from build123d import *

# Parameters (mm, degrees)
SKETCH_1_W             = 50
SKETCH_1_H             = 136
EXTRUDE_1_DEPTH        = 2
SKETCH_3_R             = 1.525
CUT_EXTRUDE_1_DEPTH    = 10
CUT_EXTRUDE_2_DEPTH    = 22
PATTERN_LINEAR_1_COUNT = 5
PATTERN_LINEAR_1_PITCH = 14
MIRROR_2_COPY_1_DEPTH  = 22
MIRROR_2_COPY_2_DEPTH  = 22
MIRROR_2_COPY_3_DEPTH  = 22
MIRROR_2_COPY_4_DEPTH  = 22
MIRROR_2_COPY_5_DEPTH  = 22
FILLET_1_R             = 2


with BuildPart() as part:
    # 草图1 → 凸台-拉伸1 (new body)
    with BuildSketch(Plane.XY):
        Rectangle(SKETCH_1_W, SKETCH_1_H)
    extrude(amount=EXTRUDE_1_DEPTH)

    # 草图3 → 切除-拉伸1 (cut)
    with BuildSketch(Plane(origin=(0, 0, 0), x_dir=(-1, 0, 0), z_dir=(0, 0, -1))):
        with Locations((-13, 65)):
            Circle(SKETCH_3_R)
        with Locations((7, 65)):
            Circle(SKETCH_3_R)
    cut_extrude_1 = extrude(amount=-CUT_EXTRUDE_1_DEPTH, mode=Mode.SUBTRACT)

    # 镜向1: 切除-拉伸1 across plane
    add(cut_extrude_1.mirror(Plane.ZX), mode=Mode.SUBTRACT)

    # 草图4 → 切除-拉伸2 (cut)
    with BuildSketch(Plane(origin=(0, 0, 0), x_dir=(-1, 0, 0), z_dir=(0, 0, -1))):
        with BuildLine():
            Line((16, -5), (-16, -5))
            ThreePointArc((-16, -5), (-21, 0), (-16, 5))
            Line((-16, 5), (16, 5))
            ThreePointArc((16, 5), (21, 0), (16, -5))
        make_face()
    cut_extrude_2 = extrude(amount=-CUT_EXTRUDE_2_DEPTH, mode=Mode.SUBTRACT)

    # 阵列(线性)1: 切除-拉伸2 ×5
    with Locations(*[(0, -i * PATTERN_LINEAR_1_PITCH, 0) for i in range(1, PATTERN_LINEAR_1_COUNT)]):
        add(cut_extrude_2, mode=Mode.SUBTRACT)

    # 镜向2 copy 1 sketch → 镜向2 copy 1 (cut)
    with BuildSketch(Plane(origin=(0, 14, 0), x_dir=(-1, 0, 0), z_dir=(0, 0, -1))):
        with BuildLine():
            Line((16, 5), (-16, 5))
            ThreePointArc((-16, 5), (-21, 0), (-16, -5))
            Line((-16, -5), (16, -5))
            ThreePointArc((16, -5), (21, 0), (16, 5))
        make_face()
    extrude(amount=-MIRROR_2_COPY_1_DEPTH, mode=Mode.SUBTRACT)

    # 镜向2 copy 2 sketch → 镜向2 copy 2 (cut)
    with BuildSketch(Plane(origin=(0, 28, 0), x_dir=(-1, 0, 0), z_dir=(0, 0, -1))):
        with BuildLine():
            Line((16, 5), (-16, 5))
            ThreePointArc((-16, 5), (-21, 0), (-16, -5))
            Line((-16, -5), (16, -5))
            ThreePointArc((16, -5), (21, 0), (16, 5))
        make_face()
    extrude(amount=-MIRROR_2_COPY_2_DEPTH, mode=Mode.SUBTRACT)

    # 镜向2 copy 3 sketch → 镜向2 copy 3 (cut)
    with BuildSketch(Plane(origin=(0, 42, 0), x_dir=(-1, 0, 0), z_dir=(0, 0, -1))):
        with BuildLine():
            Line((16, 5), (-16, 5))
            ThreePointArc((-16, 5), (-21, 0), (-16, -5))
            Line((-16, -5), (16, -5))
            ThreePointArc((16, -5), (21, 0), (16, 5))
        make_face()
    extrude(amount=-MIRROR_2_COPY_3_DEPTH, mode=Mode.SUBTRACT)

    # 镜向2 copy 4 sketch → 镜向2 copy 4 (cut)
    with BuildSketch(Plane(origin=(0, 56, 0), x_dir=(-1, 0, 0), z_dir=(0, 0, -1))):
        with BuildLine():
            Line((16, 5), (-16, 5))
            ThreePointArc((-16, 5), (-21, 0), (-16, -5))
            Line((-16, -5), (16, -5))
            ThreePointArc((16, -5), (21, 0), (16, 5))
        make_face()
    extrude(amount=-MIRROR_2_COPY_4_DEPTH, mode=Mode.SUBTRACT)

    # 镜向2 copy 5 sketch → 镜向2 copy 5 (cut)
    with BuildSketch(Plane(origin=(0, 0, 0), x_dir=(-1, 0, 0), z_dir=(0, 0, -1))):
        with BuildLine():
            Line((16, 5), (-16, 5))
            ThreePointArc((-16, 5), (-21, 0), (-16, -5))
            Line((-16, -5), (16, -5))
            ThreePointArc((16, -5), (21, 0), (16, 5))
        make_face()
    extrude(amount=-MIRROR_2_COPY_5_DEPTH, mode=Mode.SUBTRACT)

    # 圆角1
    fillet_1_edges = [part.edges().sort_by_distance(p)[0] for p in [
        (25, -68, 1),
        (-25, -68, 1),
        (-25, 68, 1),
        (25, 68, 1),
    ]]
    fillet(fillet_1_edges, radius=FILLET_1_R)


solid = part.part
Geometry: final body of the model. Coordinates: model frame, mm. A direction names the side the tool comes from. Give positions to 0.01 mm unless a question says otherwise; leave off trailing zeros. Write each loop counter-clockwise with the first axis right and the second up, starting at its lowest first coordinate (ties: lowest second). Pieces come first, ordered by that corner, then holes.
(1) Ray query, line 1 (X direction, y = -65, z = 0.8) (3 decimals); line 2 (X direction, y = -14, z = 0.6); line 3 (X direction, y = -18, z = 0.5). Return the intervals inside material, ascending.
(2) Access query for faces 1 (the flat face through (-3.8, 5.4, 0)), 2 (the cylindrical face through (21, -28, 1)). Directions: +Z, -Z, +X, -X, +Y, -Y. A direction counts if a zero-diameter tool reaches every point of the face in a straight line with its end or side. Return the directions, or none.
(3) Cut plane B-B, the plane x = 13. Give the number of separate pieces and of enclosed holes in the cut face, then the cut area to 3 significant figures.
(4) Cut plane A-A, the plane y = -25. Return loops of the section in (x, z), then the cut area to 3 significant figures.
Values follow:
1. line 1: x = -25 to -8.525, -5.475 to 11.475, 14.525 to 25
1. line 2: x = -25 to -21, 21 to 25
1. line 3: x = -25 to -19, 19 to 25
2. face 1: -Z, +X, -X, +Y, -Y
2. face 2: +Z, -Z
3. separate pieces: 12
3. enclosed holes: 0
3. area: 79.8 mm2
4. outline: (-25, 0) - (-20, 0) - (-20, 2) - (-25, 2) - close; (20, 0) - (25, 0) - (25, 2) - (20, 2) - close
4. area: 20.0 mm2
